from build123d import *

# Parameters (mm, degrees)
SKETCH_1_R          = 1.5
SKETCH_1_W          = 63.4
SKETCH_1_H          = 12.5
EXTRUDE_1_DEPTH     = 14
SKETCH_2_W          = 63.4
SKETCH_2_H          = 10
CUT_EXTRUDE_1_DEPTH = 8.6


with BuildPart() as part:
    # Эскиз1 → Бобышка-Вытянуть1 (new body)
    with BuildSketch(Plane(origin=(0, 0, 0), x_dir=(1, 0, 0), z_dir=(0, 1, 0))):
        with BuildLine():
            Line((0, 0), (1, 0))
            Line((1, 0), (1, 10.5))
            ThreePointArc((1, 10.5), (-3.5, 15), (1, 19.5))
            Line((1, 19.5), (73, 19.5))
            ThreePointArc((73, 19.5), (77.5, 15), (73, 10.5))
            Line((73, 10.5), (73, 0))
            Line((73, 0), (74, 0))
            Line((74, 0), (74, -10))
            Line((74, -10), (0, -10))
            Line((0, -10), (0, 0))
        make_face()
        with Locations(Location((1, 15, 0), (0, 0, 270))):
            Circle(SKETCH_1_R, mode=Mode.SUBTRACT)
        with Locations(Location((73, 15, 0), (0, 0, 270))):
            Circle(SKETCH_1_R, mode=Mode.SUBTRACT)
        with Locations((37, 6.25)):
            Rectangle(SKETCH_1_W, SKETCH_1_H, mode=Mode.SUBTRACT)
    extrude(amount=EXTRUDE_1_DEPTH)

    # Эскиз2 → Вырез-Вытянуть1 (cut)
    with BuildSketch(Plane.XZ):
        with Locations((37, 5)):
            Rectangle(SKETCH_2_W, SKETCH_2_H)
    extrude(amount=-CUT_EXTRUDE_1_DEPTH, mode=Mode.SUBTRACT)


solid = part.part
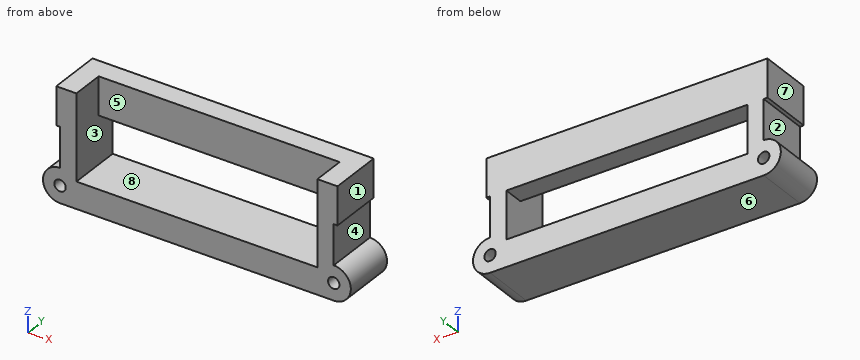
Read the model definition and answer for the solid it produces. Units are mm, in the model's axes. Face numbers are marked on the shaded views. A direction names the side the tool comes from. Give positions to 0.01 mm unless a question says otherwise; leave off trailing zeros. Write each loop counter-clockwise with the first axis right and the second up, starting at its lowest first coordinate (ties: lowest second). Pieces come first, ordered by that corner, then holes. Notation, with made-up numbers: (73.5, 49.5) - (110.5, 49.5) arc R26 cw to (110.5, 85.5) - close; hole circle Ø2 at (46, 48). An arc over 180 degrees is marked (long way). Return JSON: item names as keys, results as strings.
Q1. Given P1, Ø2.5, axis at x = 73, z = -15, coming from the -Y side; P2, Ø8, axis at x = 25.5, z = 3.5, coming from the -Y side; P3, Ø7, axis at y = 7, z = 4, coming from the -X side; P4, Ø5, axis at y = 9, z = -3.5, coming from the +X side, each flat-ended and moving along its own axis, determine where each tip first touches the part or whether it passes through.
Reply:
{"P1": "through", "P2": "y = 8.6", "P3": "x = 0", "P4": "x = 73"}
Q2. A cutting plane is placed at A-A, the plane y = 11.25. Determine the outline of the cut face in (x, z).
Reply:
{"outline": "(0, 0) - (1, 0) - (1, -10.5) arc R4.5 ccw to (1, -19.5) - (73, -19.5) arc R4.5 ccw to (73, -10.5) - (73, 0) - (74, 0) - (74, 10) - (0, 10) - close; hole circle Ø3 at (1, -15); hole (5.3, -12.5) - (68.7, -12.5) - (68.7, 0) - (5.3, 0) - close; hole circle Ø3 at (73, -15)"}
Q3. For the marked faces 1, 2, 3, 4 and 5, determine the directions among +Z, -Z, +X, -X, +Y, -Y from which every point of the face is accessible in a straight line to the end or side of a thin tool.
Reply:
{"face 1": "+Z, +X, +Y, -Y", "face 2": "-X, +Y, -Y", "face 3": "-Y", "face 4": "+X, +Y, -Y", "face 5": "+Z, -Y"}
Q4. A cutting plane is placed at D-D, the plane y = 4. Determine the outline of the cut face in (x, z).
Reply:
{"outline": "(0, 0) - (1, 0) - (1, -10.5) arc R4.5 ccw to (1, -19.5) - (73, -19.5) arc R4.5 ccw to (73, -10.5) - (73, 0) - (74, 0) - (74, 10) - (68.7, 10) - (68.7, -12.5) - (5.3, -12.5) - (5.3, 10) - (0, 10) - close; hole circle Ø3 at (1, -15); hole circle Ø3 at (73, -15)"}
Q5. Consider line 1 along X through (y, z) = (8.5, -15); line 2 along X through (y, z) = (4, 2); line 3 along X through (y, z) = (1.25, -4). Determine where each line is inside the solid, lowest interval first. Write a range as [from, to].
Reply:
{"line 1": "[-3.5, -0.5], [2.5, 71.5], [74.5, 77.5]", "line 2": "[0, 5.3], [68.7, 74]", "line 3": "[1, 5.3], [68.7, 73]"}
Q6. A cutting plane is placed at B-B, the plane x = 11.5. Determine the outline of the cut face in (y, z).
Reply:
{"outline": "(0, -19.5) - (14, -19.5) - (14, -12.5) - (0, -12.5) - close; (8.6, 0) - (14, 0) - (14, 10) - (8.6, 10) - close"}
Q7. For a pull along Z with two mould halves and no side action, classify the marked faces 6, 7 and 8 as released by +Z, released by -Z, zero draft, split by the parting line, or undercut.
Reply:
{"face 6": "released by -Z", "face 7": "zero draft", "face 8": "undercut"}
Q8. A cutting plane is placed at C-C, the plane z = -15. Determine the outline of the cut face in (x, y), and give its area (3 significant figures).
Reply:
{"outline": "(-3.5, 0) - (-0.5, 0) - (-0.5, 14) - (-3.5, 14) - close; (2.5, 0) - (71.5, 0) - (71.5, 14) - (2.5, 14) - close; (74.5, 0) - (77.5, 0) - (77.5, 14) - (74.5, 14) - close", "area": "1,050 mm²"}
